from build123d import *

# Parameters (mm, degrees)
BOSS_EXTRU_2_DEPTH           = 13.8
ENL_V_MAT_EXTRU_1_DEPTH      = 33.759120867
ENL_V_MAT_EXTRU_1_DEPTH_BACK = 13.8
CONG_1_R                     = 1.2
ENL_V_MAT_EXTRU_4_DEPTH      = 33.759120867
ENL_V_MAT_EXTRU_4_DEPTH_BACK = 13.8
CONG_2_R                     = 1.2
BOSS_EXTRU_4_DEPTH           = 4.8
BOSS_EXTRU_5_DEPTH           = 2.4
ESQUISSE8_R                  = 3
ENL_V_MAT_EXTRU_5_DEPTH      = 12


with BuildPart() as part:
    # Esquisse1 → Boss.-Extru.2 (new body)
    with BuildSketch(Plane.XY):
        Polygon((-8.4, 14.4), (-13.2, 14.4), (-13.2, -14.4), (-8.4, -14.4), (-8.4, -20.4), (-6, -20.4), (-6, -14.4), (13.2, -14.4), (13.2, 14.4), (-6, 14.4), (-6, 20.4), (-8.4, 20.4), align=None)
    extrude(amount=BOSS_EXTRU_2_DEPTH)

    # Esquisse3 → Enlèv. mat.-Extru.1 (cut, two sides: drawn at the far end of the back side and taken through both)
    with BuildSketch(Plane.ZY.offset(8.4).offset(-ENL_V_MAT_EXTRU_1_DEPTH_BACK)):
        with BuildLine():
            Line((5.7, 113.592547743), (5.7, 20.4))
            Line((5.7, 20.4), (5.7, 16.8))
            ThreePointArc((5.7, 16.8), (6.9, 15.6), (8.1, 16.8))
            Line((8.1, 16.8), (8.1, 20.4))
            Line((8.1, 20.4), (8.1, 113.592547743))
            Line((8.1, 113.592547743), (8.1, 299.97764323))
            Line((8.1, 299.97764323), (5.7, 299.97764323))
            Line((5.7, 299.97764323), (5.7, 113.592547743))
        make_face()
    extrude(amount=ENL_V_MAT_EXTRU_1_DEPTH + ENL_V_MAT_EXTRU_1_DEPTH_BACK, mode=Mode.SUBTRACT)

    # Congé1
    cong_1_edges = [part.edges().sort_by_distance(p)[0] for p in [
        (-7.2, 20.4, 0),
        (-7.2, 20.4, 13.8),
    ]]
    fillet(cong_1_edges, radius=CONG_1_R)

    # Esquisse5 → Enlèv. mat.-Extru.4 (cut, two sides: drawn at the far end of the back side and taken through both)
    with BuildSketch(Plane.ZY.offset(8.4).offset(-ENL_V_MAT_EXTRU_4_DEPTH_BACK)):
        with BuildLine():
            Line((5.7, -16.8), (5.7, -20.4))
            Line((5.7, -20.4), (8.1, -20.4))
            Line((8.1, -20.4), (8.1, -16.8))
            ThreePointArc((8.1, -16.8), (6.9, -15.6), (5.7, -16.8))
        make_face()
    extrude(amount=ENL_V_MAT_EXTRU_4_DEPTH + ENL_V_MAT_EXTRU_4_DEPTH_BACK, mode=Mode.SUBTRACT)

    # Congé2
    cong_2_edges = [part.edges().sort_by_distance(p)[0] for p in [
        (-7.2, -20.4, 0),
        (-7.2, -20.4, 13.8),
    ]]
    fillet(cong_2_edges, radius=CONG_2_R)

    # Esquisse6 → Boss.-Extru.4 (add)
    with BuildSketch(Plane.ZY.offset(13.2)):
        with BuildLine():
            Line((3.3, -1.960815773), (3.3, -0.355303277))
            ThreePointArc((3.3, -0.355303277), (1.40200229, 1.026689827), (0, 2.909955561))
            Line((0, 2.909955561), (0, 10.256412893))
            ThreePointArc((0, 10.256412893), (6.9, 14.4), (13.8, 10.256412893))
            Line((13.8, 10.256412893), (13.8, 2.909955561))
            ThreePointArc((13.8, 2.909955561), (12.39799771, 1.026689827), (10.5, -0.355303277))
            Line((10.5, -0.355303277), (10.5, -1.960815773))
            ThreePointArc((10.5, -1.960815773), (6.9, -5.560815773), (3.3, -1.960815773))
        make_face()
    extrude(amount=BOSS_EXTRU_4_DEPTH)

    # Esquisse7 → Boss.-Extru.5 (add)
    with BuildSketch(Plane.ZY.offset(18)):
        with BuildLine():
            Line((5.1, -1.960815773), (5.1, 1.500148416))
            ThreePointArc((5.1, 1.500148416), (7.011460398, 11.971564485), (8.7, 1.461898964))
            Line((8.7, 1.461898964), (8.7, -1.960815773))
            ThreePointArc((8.7, -1.960815773), (6.9, -3.760815773), (5.1, -1.960815773))
        make_face()
    extrude(amount=BOSS_EXTRU_5_DEPTH)

    # Esquisse8 → Enlèv. mat.-Extru.5 (cut)
    with BuildSketch(Plane.ZY.offset(20.4)):
        with Locations((6.954089459, 6.571869256)):
            Circle(ESQUISSE8_R)
    extrude(amount=-ENL_V_MAT_EXTRU_5_DEPTH, mode=Mode.SUBTRACT)


solid = part.part
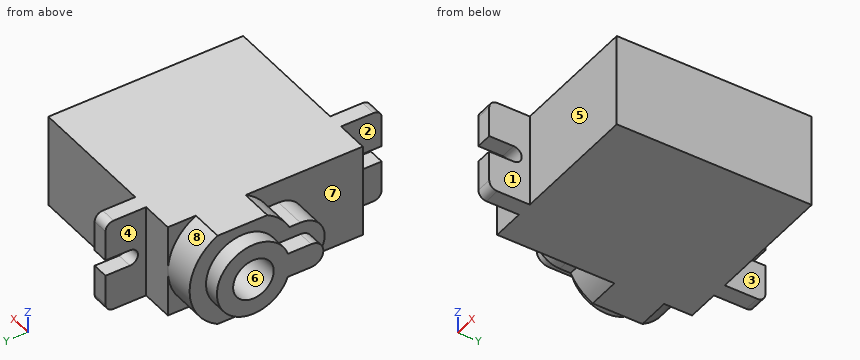
Model file for the job. Use its own axes, mm. Face numbers are marked on the shaded views. A direction names the side the tool comes from. Give positions to 0.01 mm unless a question says otherwise; leave off trailing zeros. Order: outer loops, then holes, each group sorted by start corner. A loop starts at its lowest first (then second) coordinate and runs counter-clockwise, first axis right, second up. Notation, with made-up numbers: M 55.25,56 L 83.25,56 A29 cw 83.25,88 Z; hole C 71.5,-21 d3. An arc over 180 degrees is marked long. Put each result on its own line as item: value. Start each with the question number.
(1) Band-saw the part on A-A on x = -9.5. Give the cut face in (y, z).
(2) Pull direction Y, two halves, no side cores. Call the marked faces 5, 6, 7 and 8: released by +Y, released by -Y, zero draft, split by the parting line, or undercut.
(3) Band-saw the part on D-D on x = -17. Give the cut face in (y, z), then the cut area to 3 significant figures.
(4) Drill centre lines: L1, parallel to X at y = 13, z = 11.5; L2, parallel to Y at x = 0, z = 11; L3, parallel to X at y = 3.5, z = 1.5. Where is each one in solid material? Low to high. Write a range as [from, to].
(5) Band-saw the part on B-B on y = 8. Give the cut face in (x, z), then the cut area to 3 significant figures.
(6) Pin check, flat tips, straight feed: pin 1 Ø0.7 at (x, y) = (-19.5, 0.5) entering from +Z; pin 2 Ø1.5 at (y, z) = (-16, 7.5) entering from -X; pin 3 Ø1.5 at (x, y) = (2, 16) entering from -Z; pin 4 Ø4 at (x, z) = (8, 10) entering from +Y. Stop position of each tip, or through.
(7) Tool access for the marked faces 1, 2, 3 and 4: list every direction of +Z, -Z, +X, -X, +Y, -Y with a clear straight run to the whole face (end or side of a thin tool).
(8) Band-saw the part on C-C on x = 8. Give the cut face in (y, z).
Results below:
1. outline: M -14.4,0 L 14.4,0 L 14.4,13.8 L -14.4,13.8 Z; hole C 6.57,6.95 d6
2. face 5: released by -Y
2. face 6: undercut
2. face 7: zero draft
2. face 8: released by +Y
3. outline: M -1.96,3.3 L -0.36,3.3 A7.82 ccw 2.91,0 L 10.26,0 A7.82 ccw 10.26,13.8 L 2.91,13.8 A7.82 ccw -0.36,10.5 L -1.96,10.5 A3.6 ccw Z; hole C 6.57,6.95 d6
3. area: 182 mm2
4. L1: x = [-13.2, 13.2]
4. L2: y = [-14.4, 14.4]
4. L3: x = [-18, 13.2]
5. outline: M -20.4,1.75 L -18,1.75 L -18,0 L 13.2,0 L 13.2,13.8 L -18,13.8 L -18,12.16 L -20.4,12.16 L -20.4,9.59 L -8.4,9.59 L -8.4,4.32 L -20.4,4.32 Z
5. area: 392 mm2
6. pin 1: stops at z = 8.7
6. pin 2: stops at x = -8.4
6. pin 3: passes through
6. pin 4: stops at y = 14.4
7. face 1: +Z, -Z, +X, -Y
7. face 2: +Z, -Z, -X, -Y
7. face 3: +Z, -Z, +X, +Y
7. face 4: +Z, -Z, -X, +Y
8. outline: M -14.4,0 L 14.4,0 L 14.4,13.8 L -14.4,13.8 Z
